Autodesk Inventor part; units mm, degrees
ref_plane "YZ Plane" through (0, 0, 0) normal (1, 0, 0) x (0, 1, 0)
ref_plane "XZ Plane" through (0, 0, 0) normal (0, 1, 0) x (-1, 0, 0)
ref_plane "XY Plane" through (0, 0, 0) normal (0, 0, 1) x (1, 0, 0)
sketch "Sketch1" plane through (0, 0, 0) normal (0, 1, 0) x (-1, 0, 0)
  arc A0 (-2.2913, 1) -> (2.2913, 1) centre (0, 0) ccw
  circle A1 centre (0, 0) radius 3.088
  line L0 (2.6552, 1.6) -> (-2.6552, 1.6)
  line L1 (-2.6411, 1.6) -> (2.6552, 1.6)
  line L2 (2.2913, 1) -> (-2.2913, 1)
  circle A2 centre (0, 0) radius 7.5
  line L3 (7.5, 0) -> (7.5, 50)
  line L4 (7.5, 50) -> (-7.5, 50)
  line L5 (-7.5, 50) -> (-7.5, 0)
  point P0 (2.6411, 1.6)
  point P1 (-2.6411, 1.6)
  dimension "d1" = 15
  dimension "d2" = 50
extrude "Extrusion1" add sketch "Sketch1" along normal blind 10 contours A1 L0 | A2 picked at (0.7371, 1.7852)
extrude "Extrusion2" add sketch "Sketch1" along normal blind 5 contours A2 L5 L4 L3
chamfer "Chamfer1" distance 5 angle 45 2 edges at (-7.5, 2.5, 50) (7.5, 2.5, 50)
sketch "Sketch3" plane through (0, 0, 0) normal (0, -1, 0) x (1, 0, 0)
  line L0 (-5, 42) -> (0, 47)
  line L1 (-2.5, 50) -> (-7.5, 45)
  line L2 (0, 47) -> (5, 42)
  line L3 (5, 42) -> (-5, 42)
  line L4 (-5, 42) -> (-5, 12)
  line L5 (5, 12) -> (5, 42)
  line L6 (-2.5, 50) -> (2.5, 50)
  line L7 (-5, 12) -> (-5, 5.5902)
  arc A0 (7.5, 0) -> (-7.5, 0) centre (0, 0) ccw
  line L8 (5, 12) -> (5, 5.5902)
  circle A1 centre (0, 0) radius 7.5
  line L9 (5, 12) -> (-5, 12)
  dimension "d13" = 10
  dimension "d14" = 30
  dimension "d15" = 3
extrude "Extrusion3" cut sketch "Sketch3" against normal blind 5.5 contours L0 L2 L3 | L3 L5 L9 L4
chamfer "Chamfer2" distance 5 angle 45 2 edges at (-5, 2.5, 12) (5, 2.5, 12)
properties part number "StepMotorTest"
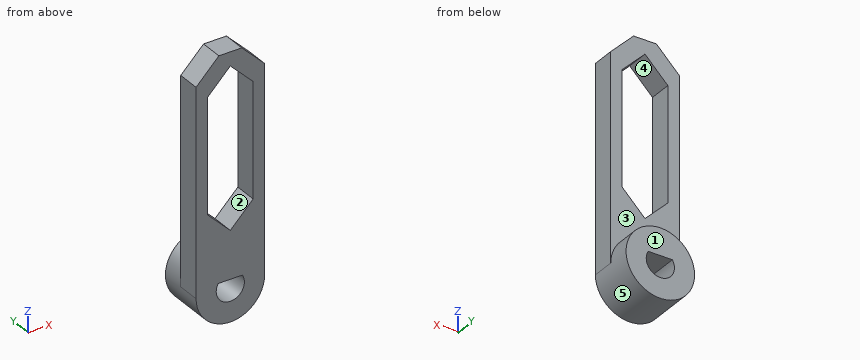
Could you check a few things on this model? Use its own coordinates, in mm. Face numbers are marked on the shaded views. A direction names the side the tool comes from. Coordinates: 2 decimals unless noted, no trailing zeros. Order: outer loops, then holes, each group sorted by start corner. A loop starts at its lowest first (then second) coordinate and runs counter-clockwise, first axis right, second up. Notation, with made-up numbers: (36, 67) - (64, 67) arc R27 ccw to (64, 94) - close; hole circle Ø4 at (24.25, 73.5). An arc over 180 degrees is marked (long way). Answer in a Markdown table with one row per item. Add a question column.
(1) On a 3-axis mill with a long thin cutter (end or side, diameter ignored), from which of +Z, -Z, +X, -X, +Y, -Y can I reach the whole of each face in a straight line? I mean the marked faces 1 and 2. Say none if no direction works.
(2) I need wall thicknesses on L1, parallel to Z at x = 2.75, y = 2; L2, parallel to X at y = 1.5, z = 42; L3, parallel to Z at x = 1.5, y = 1. Which ranges of each line are inside material? Lowest first, please.
(3) If we section it at B-B, the plane x = 1.25: Please give me the cut outline in (y, z).
(4) If we mould it in two halves opening along X, with no side actions, what happens to the marked faces 3, 4 and 5? For each: released by +X, released by -X, zero draft, split by the parting line, or undercut.
(5) If we section it at C-C, the plane y = 5.75: Please give me the cut outline in (x, z), then the cut area to 3 significant figures.
(6) If we section it at A-A, the plane z = 27.5: Please give me the cut outline in (x, y).
(7) Will these pins go through, and if not, where does the flat tip stop? pin 1 (1 mm diameter, centred on y = 6.5, z = 40, fed in from +X); pin 2 (1 mm diameter, centred on x = 0.5, y = 6.5, fed in from +Z).
(8) If we section it at D-D, the plane z = 6.5: Please give me the cut outline in (x, y).
Results are:
| question | item | result |
|---|---|---|
| 1 | face 1 | +Z, -Z, +X, -X, +Y |
| 1 | face 2 | +Y, -Y |
| 2 | L1 | z = -6.98 to -1.4, 1.4 to 14.75, 44.25 to 49.75 |
| 2 | L2 | x = -7.5 to -5, 5 to 7.5 |
| 2 | L3 | z = -7.35 to -2.7, 1.6 to 13.5, 45.5 to 50 |
| 3 | outline | (0, -7.4) - (10, -7.4) - (10, -2.82) - (0, -2.82) - close; (0, 1.6) - (10, 1.6) - (10, 7.4) - (5, 7.4) - (5, 13.25) - (0, 13.25) - close; (0, 45.75) - (5, 45.75) - (5, 50) - (0, 50) - close |
| 4 | face 3 | zero draft |
| 4 | face 4 | undercut |
| 4 | face 5 | split by the parting line |
| 5 | outline | circle Ø15 at (0, 0); hole (-2.64, 1.6) arc R3.09 ccw (long way) to (2.64, 1.6) - close |
| 5 | area | 152 mm2 |
| 6 | outline | (-7.5, 0) - (-5, 0) - (-5, 5) - (-7.5, 5) - close; (5, 0) - (7.5, 0) - (7.5, 5) - (5, 5) - close |
| 7 | pin 1 | passes through |
| 7 | pin 2 | stops at z = 7.5 |
| 8 | outline | (-7.5, 0) - (7.5, 0) - (7.5, 5) - (3.74, 5) - (3.74, 10) - (-3.74, 10) - (-3.74, 5) - (-7.5, 5) - close |
